Design review of the part built by this model. Coordinates are the model's own, in mm. Face numbers are marked on the shaded views. Give positions to 0.01 mm unless a question says otherwise; leave off trailing zeros. Loops run counter-clockwise (first coordinate to the right, second up) from the corner with the lowest first, then second, coordinate; pieces in that order, holes last. Notation, with made-up numbers: (69, -15) -> (97, -15) arc R21 ccw to (97, 5) -> close; hole circle Ø8 at (-32, -18). An arc over 180 degrees is marked (long way). Answer in a Markdown table with one row per item. Add a question column.
(1) For line 1 (X direction, y = 13, z = 0); line 2 (X direction, y = 6, z = 0.55); line 3 (Z direction, x = 1.75, y = 9), list the stretches that pass through material, from the lowest coordinate up.
(2) For pin 1 (3.5 mm diameter, centred on x = 0, z = 0, fed in from -Y); pin 2 (1 mm diameter, centred on y = 18, z = -2, fed in from -X), all flat-tipped, find the tip position at first contact; note any pin that passes through.
(3) Draft analysis for pull direction Z (two halves, no side actions). For the marked faces 1, 2 and 3, state which applies: +Z half, -Z half, draft (parallel to the pull), parting line (faces both ways), or undercut.
(4) Consider section B-B on x = 0. Write out the cut boundary in (y, z).
(5) Consider section A-A on y = 6. Write out the cut boundary in (x, z), then the cut area to 3 significant figures.
from build123d import *

# Parameters (mm, degrees)
SKETCH_1_R      = 2
EXTRUDE_1_DEPTH = 50


with BuildPart() as part:
    # 草图1 → 凸台-拉伸1 (new body)
    with BuildSketch(Plane(origin=(0, 0, 0), x_dir=(1, 0, 0), z_dir=(0, 1, 0))):
        Polygon((1.703183294, -2.95), (3.406366588, 0), (1.703183294, 2.95), (-1.703183294, 2.95), (-3.406366588, 0), (-1.703183294, -2.95), align=None)
        with Locations(Location((0, 0, 0), (0, 0, 270))):
            Circle(SKETCH_1_R, mode=Mode.SUBTRACT)
    extrude(amount=EXTRUDE_1_DEPTH)

    # 草图3 → 切除-旋转1 (revolve, cut)
    with BuildSketch(Plane.XY, mode=Mode.PRIVATE) as cut_revolve_1_sk:
        Polygon((6.978635767, 3.2), (1.2, -1), (6.978635767, -1), align=None)
    cut_revolve_1 = revolve(cut_revolve_1_sk.sketch.rotate(Axis((0, 59.182101856, 0), (0, -1, 0)), 90), axis=Axis((0, 59.182101856, 0), (0, -1, 0)), mode=Mode.SUBTRACT)

    # 镜向1: 切除-旋转1 across plane
    add(cut_revolve_1.mirror(Plane.ZX.offset(25)), mode=Mode.SUBTRACT)


solid = part.part
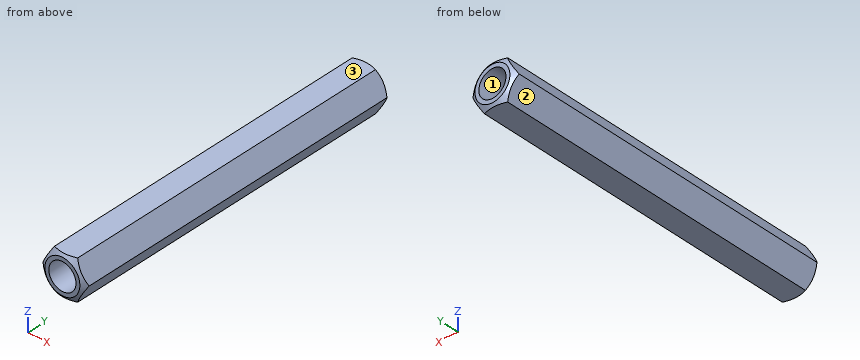
Values follow:
| question | item | result |
|---|---|---|
| 1 | line 1 | -3.41 to -2, 2 to 3.41 |
| 1 | line 2 | -3.09 to -1.92, 1.92 to 3.09 |
| 1 | line 3 | -2.87 to -0.97, 0.97 to 2.87 |
| 2 | pin 1 | through |
| 2 | pin 2 | x = -2.54 |
| 3 | face 1 | undercut |
| 3 | face 2 | -Z half |
| 3 | face 3 | +Z half |
| 4 | outline | (0, -2.58) -> (0.27, -2.95) -> (49.73, -2.95) -> (50, -2.58) -> (50, -2) -> (0, -2) -> close; (0, 2) -> (50, 2) -> (50, 2.58) -> (49.73, 2.95) -> (0.27, 2.95) -> (0, 2.58) -> close |
| 5 | outline | (-3.41, 0) -> (-1.7, -2.95) -> (1.7, -2.95) -> (3.41, 0) -> (1.7, 2.95) -> (-1.7, 2.95) -> close; hole circle Ø4 at (0, 0) |
| 5 | area | 17.6 mm2 |
